```python
from build123d import *

# Parameters (mm, degrees)
SKETCH1_W           = 38.1
SKETCH1_H           = 38.1
SKETCH1_W_2         = 34.925
SKETCH1_H_2         = 34.925
BOSS_EXTRUDE1_DEPTH = 762
SKETCH2_R           = 2.5527
CUT_EXTRUDE1_DEPTH  = 39.1
SKETCH3_R           = 2.5527
SKETCH3_R_2         = 1.5875
CUT_EXTRUDE2_DEPTH  = 39.1
SKETCH4_R           = 14.2875
SKETCH4_R_2         = 2.5527
CUT_EXTRUDE3_DEPTH  = 39.1


with BuildPart() as part:
    # Sketch1 → Boss-Extrude1 (new body)
    with BuildSketch(Plane(origin=(0, 0, 0), x_dir=(1, 0, 0), z_dir=(0, 1, 0))):
        Rectangle(SKETCH1_W, SKETCH1_H)
        Rectangle(SKETCH1_W_2, SKETCH1_H_2, mode=Mode.SUBTRACT)
    extrude(amount=BOSS_EXTRUDE1_DEPTH)

    # Sketch2 → Cut-Extrude1 (cut, through all)
    with BuildSketch(Plane.XY.offset(19.05)):
        with Locations((0, 76.2)):
            Circle(SKETCH2_R)
        with Locations((0, 95.25)):
            Circle(SKETCH2_R)
        with Locations((0, 114.3)):
            Circle(SKETCH2_R)
        with Locations((0, 133.35)):
            Circle(SKETCH2_R)
        with Locations((9.525, 104.775)):
            Circle(SKETCH2_R)
    extrude(amount=-CUT_EXTRUDE1_DEPTH, mode=Mode.SUBTRACT)

    # Sketch3 → Cut-Extrude2 (cut, through all)
    with BuildSketch(Plane(origin=(19.05, 0, 0), x_dir=(0, 0, -1), z_dir=(1, 0, 0))):
        with Locations((0, 76.2)):
            Circle(SKETCH3_R)
        with Locations((0, 95.25)):
            Circle(SKETCH3_R)
        with Locations((0, 114.3)):
            Circle(SKETCH3_R)
        with Locations((0, 225.425)):
            Circle(SKETCH3_R_2)
        with Locations((0, 187.325)):
            Circle(SKETCH3_R_2)
        with Locations((0, 752.475)):
            Circle(SKETCH3_R)
        with Locations((0, 733.425)):
            Circle(SKETCH3_R)
    extrude(amount=-CUT_EXTRUDE2_DEPTH, mode=Mode.SUBTRACT)

    # Sketch4 → Cut-Extrude3 (cut, through all)
    with BuildSketch(Plane(origin=(19.05, 0, 0), x_dir=(0, 0, -1), z_dir=(1, 0, 0))):
        with Locations((0, 31.75)):
            Circle(SKETCH4_R)
        with Locations((-11.90625, 52.372229928)):
            Circle(SKETCH4_R_2)
        with Locations((11.90625, 52.372229928)):
            Circle(SKETCH4_R_2)
        with Locations((11.90625, 11.127770072)):
            Circle(SKETCH4_R_2)
        with Locations((-11.90625, 11.127770072)):
            Circle(SKETCH4_R_2)
    extrude(amount=-CUT_EXTRUDE3_DEPTH, mode=Mode.SUBTRACT)


solid = part.part
```
For this review, take the finished solid that the model builds, in its own axes (mm). A direction names the side the tool comes from. Round coordinates to 2 decimals unless told otherwise and drop trailing zeros. Loops run counter-clockwise (first coordinate to the right, second up) from the corner with the lowest first, then second, coordinate; pieces in that order, holes last.
Q1. Add section A-A on y = 172.5. Write out the cut boundary in (x, z), plus the area to 3 significant figures.
Result sheet:
outline: (-19.05, -19.05) - (19.05, -19.05) - (19.05, 19.05) - (-19.05, 19.05) - close; hole (-17.46, -17.46) - (17.46, -17.46) - (17.46, 17.46) - (-17.46, 17.46) - close
area: 232 mm2
Q2. Machinability: for faces 4 (the face through (0, 376, 19.05)), 5 (the face through (0, 376, -17.462)), which of the approach directions +Z, -Z, +X, -X, +Y, -Y give a long, thin tool a straight path to every point of the face, cutting with its end or side? Answer none if there is none.
Result sheet:
face 4: +Z, +X, -X, +Y, -Y
face 5: +Y, -Y
Q3. Insertion check: pin 1 Ø8 at (y, z) = (733.425, 0) entering from +X. The pin has a flat end and moves straight along its axis. Give the tip position at first contact, or say it passes through.
Result sheet:
pin 1: stops at x = 19.05
Q4. Mouldability with a two-part tool opening along Y and no side actions: class faces 1 (the face through (19.05, 376, 0)), 2 (the face through (-2, 0, 18)), 3 (the face through (-18.245, 17.802, 3.097)) as +Y half, -Y half, draft (parallel to the pull), parting line (faces both ways), or undercut.
Result sheet:
face 1: draft
face 2: -Y half
face 3: undercut
Q5. To check wall thickness, follow line 1 along Z through (x, y) = (-1.5, 681); line 2 along Y through (x, z) = (0, 17.9). State the ranges of each line that lie inside material, in increasing order.
Result sheet:
line 1: z = -19.05 to -17.46, 17.46 to 19.05
line 2: y = 0 to 73.65, 78.75 to 92.7, 97.8 to 111.75, 116.85 to 130.8, 135.9 to 762
